```python
from build123d import *

# Parameters (mm, degrees)
BOSS_EXTRUDE1_DEPTH      = 1000
BOSS_EXTRUDE1_DEPTH_BACK = 1000
BOSS_EXTRUDE2_DEPTH      = 1000
BOSS_EXTRUDE2_DEPTH_BACK = 1000


with BuildPart() as part:
    # Sketch1 → Boss-Extrude1 (new, two sides: drawn at the far end of the back side and taken through both)
    with BuildSketch(Plane.XY.offset(-BOSS_EXTRUDE1_DEPTH_BACK)):
        Polygon((10, 15), (50, 15), (50, 35), (-50, 35), (-50, 15), (-10, 15), (-10, -15), (-50, -15), (-50, -35), (50, -35), (50, -15), (10, -15), align=None)
    extrude(amount=BOSS_EXTRUDE1_DEPTH + BOSS_EXTRUDE1_DEPTH_BACK)

    # Sketch2 → Boss-Extrude2 (add, two sides: drawn at the far end of the back side and taken through both)
    with BuildSketch(Plane(origin=(0, 0, 0), x_dir=(0, 0, -1), z_dir=(1, 0, 0)).offset(-BOSS_EXTRUDE2_DEPTH_BACK)):
        Polygon((10, 15.14982009), (50, 15.14982009), (50, 35.14982009), (-50, 35.14982009), (-50, 15.14982009), (-10, 15.14982009), (-10, -14.85017991), (-50, -14.85017991), (-50.000001017, -34.85017991), (49.999998983, -34.85017991), (50, -14.85017991), (10, -14.85017991), align=None)
    extrude(amount=BOSS_EXTRUDE2_DEPTH + BOSS_EXTRUDE2_DEPTH_BACK)


solid = part.part
```
Geometry check sheet. Reference: the model listing, model coordinates, mm. Round coordinates to 2 decimals unless told otherwise and drop trailing zeros. Write each loop counter-clockwise with the first axis right and the second up, starting at its lowest first coordinate (ties: lowest second). Pieces come first, ordered by that corner, then holes. Notation, with made-up numbers: (-38.5, -37.5) -> (15.5, -37.5) arc R15 cw to (15.5, -15.5) -> close; hole circle Ø2 at (47, 68.25). An arc over 180 degrees is marked (long way). Put each result on its own line as item: value.
1) Depth check by flat-ended pin: P1, Ø20, axis at x = -29.5, z = 434.5, coming from the +Y side; P2, Ø9, axis at y = 0, z = -416.5, coming from the -X side; P3, Ø9, axis at y = 4, z = -363.5, coming from the +X side. Enter the tip coordinate at first touch or a pass-through.
Recorded:
P1: stops at y = 35
P2: stops at x = -10
P3: stops at x = 10
2) Cross-section at B-B, the plane x = 396.5. Enter the section's corners in (y, z), plus the area to 3 significant figures.
Recorded:
outline: (-34.85, -50) -> (-14.85, -50) -> (-14.85, -10) -> (15.15, -10) -> (15.15, -50) -> (35.15, -50) -> (35.15, 50) -> (15.15, 50) -> (15.15, 10) -> (-14.85, 10) -> (-14.85, 50) -> (-34.85, 50) -> close
area: 4,600 mm2
3) Thickness scan on probe 1 along Y at (x, z) = (825.5, -38.5); probe 2 along X at (y, z) = (-10, 425.5). Record the ranges inside material, lowest first. Write a range as from..to.
Recorded:
probe 1: y = -34.85..-14.85, 15.15..35.15
probe 2: x = -10..10
4) Cross-section at A-A, the plane y = 3. Enter the section's corners in (x, z), plus the area to 3 significant figures.
Recorded:
outline: (-1000, -10) -> (-10, -10) -> (-10, -1000) -> (10, -1000) -> (10, -10) -> (1000, -10) -> (1000, 10) -> (10, 10) -> (10, 1000) -> (-10, 1000) -> (-10, 10) -> (-1000, 10) -> close
area: 79,600 mm2
5) Release check for a two-part mould opening along X. For faces 1 (the face through (-1000, 1, 1)), 2 (the face through (1000, 1, 1)), 3 (the face through (-1, 0, 1000)) record: pulls with the +X half, pulls with the -X half, needs draft (parallel to the pull), parting line crosses it, or undercut.
Recorded:
face 1: pulls with the -X half
face 2: pulls with the +X half
face 3: needs draft
